Can you work these out from the model? Positions are in its coordinate system, mm. A direction names the side the tool comes from. Give positions to 0.01 mm unless a question says otherwise; leave off trailing zeros. Order: outer loops, then holes, each group sorted by start corner. A loop starts at its lowest first (then second) coordinate and runs counter-clockwise, first axis right, second up.
```python
from build123d import *

# Parameters (mm, degrees)
BOSS_EXTRUDE1_DEPTH = 4
SKETCH2_R           = 3.1
CUT_EXTRUDE1_DEPTH  = 1
CUT_EXTRUDE2_START  = -1
SKETCH3_R           = 3.1
CUT_EXTRUDE2_DEPTH  = 1
SKETCH4_R           = 2.4
CUT_EXTRUDE3_DEPTH  = 84.668990672
LPATTERN1_COUNT     = 11
LPATTERN1_PITCH     = 8
CUT_EXTRUDE4_DEPTH  = 84.668990672
LPATTERN2_COUNT     = 10
LPATTERN2_PITCH     = 8


with BuildPart() as part:
    # Sketch1 → Boss-Extrude1 (new, symmetric)
    with BuildSketch(Plane(origin=(0, 0, 0), x_dir=(1, 0, 0), z_dir=(0, 1, 0))):
        with BuildLine():
            Line((0, 3.5), (80, 3.5))
            ThreePointArc((80, 3.5), (83.5, 0), (80, -3.5))
            Line((80, -3.5), (0, -3.5))
            ThreePointArc((0, -3.5), (-3.5, 0), (0, 3.5))
        make_face()
    extrude(amount=BOSS_EXTRUDE1_DEPTH, both=True)

    # Sketch2 → Cut-Extrude1 (cut)
    with BuildSketch(Plane(origin=(0, 4, 0), x_dir=(1, 0, 0), z_dir=(0, 1, 0))):
        with Locations(Location((0, 0, 0), (0, 0, 270))):
            Circle(SKETCH2_R)
    cut_extrude1 = extrude(amount=-CUT_EXTRUDE1_DEPTH, mode=Mode.SUBTRACT)

    # Sketch3 → Cut-Extrude2 (cut)
    with BuildSketch(Plane(origin=(0, -4, 0), x_dir=(-1, 0, 0), z_dir=(0, -1, 0)).offset(CUT_EXTRUDE2_START)):
        with Locations(Location((0, 0, 0), (0, 0, 270))):
            Circle(SKETCH3_R)
    cut_extrude2 = extrude(amount=CUT_EXTRUDE2_DEPTH, mode=Mode.SUBTRACT)

    # Sketch4 → Cut-Extrude3 (cut, symmetric)
    with BuildSketch(Plane(origin=(0, 0, 0), x_dir=(1, 0, 0), z_dir=(0, 1, 0))):
        with Locations(Location((0, 0, 0), (0, 0, 270))):
            Circle(SKETCH4_R)
    cut_extrude3 = extrude(amount=CUT_EXTRUDE3_DEPTH, both=True, mode=Mode.SUBTRACT)

    # LPattern1: Cut-Extrude1, Cut-Extrude2, Cut-Extrude3 ×11
    with Locations(*[(i * LPATTERN1_PITCH, 0, 0) for i in range(1, LPATTERN1_COUNT)]):
        add(cut_extrude1, mode=Mode.SUBTRACT)
        add(cut_extrude2, mode=Mode.SUBTRACT)
        add(cut_extrude3, mode=Mode.SUBTRACT)

    # Sketch5 → Cut-Extrude4 (cut, symmetric)
    with BuildSketch(Plane(origin=(0, 0, 0), x_dir=(1, 0, 0), z_dir=(0, 1, 0))):
        with BuildLine():
            Line((2.814249456, 3.1), (5.185750544, 3.1))
            ThreePointArc((5.185750544, 3.1), (5.553697029, 2.856892908), (5.474391514, 2.423076923))
            ThreePointArc((5.474391514, 2.423076923), (4.5, 0), (5.474391514, -2.423076923))
            ThreePointArc((5.474391514, -2.423076923), (5.553697029, -2.856892908), (5.185750544, -3.1))
            Line((5.185750544, -3.1), (2.814249456, -3.1))
            ThreePointArc((2.814249456, -3.1), (2.446302971, -2.856892908), (2.525608486, -2.423076923))
            ThreePointArc((2.525608486, -2.423076923), (3.5, 0), (2.525608486, 2.423076923))
            ThreePointArc((2.525608486, 2.423076923), (2.446302971, 2.856892908), (2.814249456, 3.1))
        make_face()
    cut_extrude4 = extrude(amount=CUT_EXTRUDE4_DEPTH, both=True, mode=Mode.SUBTRACT)

    # LPattern2: Cut-Extrude4 ×10
    with Locations(*[(i * LPATTERN2_PITCH, 0, 0) for i in range(1, LPATTERN2_COUNT)]):
        add(cut_extrude4, mode=Mode.SUBTRACT)


solid = part.part
```
1) Suppose I cut it at B-B (z = 0). Give the number of separate pieces and of enclosed holes in the cut face, and give its area (3 significant figures).
2) I'm going to push flat-ended pins straight in: pin 1 Ø4 at (x, z) = (32, 0) entering from -Y; pin 2 Ø4 at (x, z) = (16.5, -2.5) entering from -Y; pin 3 Ø1.5 at (x, z) = (31, -1.5) entering from +Y. Where does each tip first touch, or does it pass through?
3) Suppose I cut it at A-A (x = 64). Please give me the cut outline in (y, z), and give its area (3 significant figures).
4) We'd pull the mould along Z, two halves only. Please class faces 3 (the face through (39, 0, -3.5)), 4 (the face through (0.931, 3.507, 2.957)): +Z half, -Z half, draft (parallel to the pull), parting line (faces both ways), or undercut.
5) Which directions (+Z, -Z, +X, -X, +Y, -Y) give clear straight access to the entire face, cutting with the end or side of a thin tool? Please do faces 1 (the face through (52, 0, 3.1)), 2 (the face through (42, -3, 2)).
6) If I drill on line 1 (Z direction, x = 8, y = -3.7); line 2 (Y direction, x = 54, z = -1.75); line 3 (Z direction, x = 34, y = 1), over which ranges is the centre line in solid material (lowest first)?
Results:
1. separate pieces: 22
1. enclosed holes: 0
1. area: 163 mm2
2. pin 1: passes through
2. pin 2: stops at y = -4
2. pin 3: stops at y = 3
3. outline: (-4, -3.5) - (4, -3.5) - (4, -3.1) - (3, -3.1) - (3, -2.4) - (-3, -2.4) - (-3, -3.1) - (-4, -3.1) - close; (-4, 3.1) - (-3, 3.1) - (-3, 2.4) - (3, 2.4) - (3, 3.1) - (4, 3.1) - (4, 3.5) - (-4, 3.5) - close
3. area: 14.8 mm2
4. face 3: -Z half
4. face 4: undercut
5. face 1: +Y, -Y
5. face 2: -Y
6. line 1: z = -3.5 to -3.1, 3.1 to 3.5
6. line 2: y = -3 to 3
6. line 3: z = -3.5 to -1.33, 1.33 to 3.5
